Model file for the job. Use its own axes, mm. A direction names the side the tool comes from. Give positions to 0.01 mm unless a question says otherwise; leave off trailing zeros. Order: outer loops, then holes, each group sorted by start corner. A loop starts at its lowest first (then second) coordinate and runs counter-clockwise, first axis right, second up. Notation, with made-up numbers: (43, 52) -> (63, 52) arc R25 ccw to (63, 81) -> close; hole circle Ø9 at (18, -15.75). An arc over 180 degrees is marked (long way). Answer in a Markdown table with one row per item. Add a question column.
from build123d import *

# Parameters (mm, degrees)
SKETCH2_W           = 636
SKETCH2_H           = 753
BOSS_EXTRUDE1_DEPTH = 600
SKETCH3_W           = 600
SKETCH3_H           = 735
CUT_EXTRUDE1_DEPTH  = 600
BOSS_EXTRUDE2_START = -18
SKETCH4_W           = 600
SKETCH4_H           = 735
BOSS_EXTRUDE2_DEPTH = 9
BOSS_EXTRUDE3_START = -102
SKETCH5_W           = 636
SKETCH5_H           = 102
BOSS_EXTRUDE3_DEPTH = 18
SKETCH6_W           = 636
SKETCH6_H           = 102
BOSS_EXTRUDE4_DEPTH = 18
CUT_EXTRUDE2_REACH  = 1155.909
SKETCH7_W           = 600
SKETCH7_H           = 462


with BuildPart() as part:
    # Sketch2 → Boss-Extrude1 (new body)
    with BuildSketch(Plane.XY):
        with Locations((318, 376.5)):
            Rectangle(SKETCH2_W, SKETCH2_H)
    extrude(amount=BOSS_EXTRUDE1_DEPTH)

    # Sketch3 → Cut-Extrude1 (cut)
    with BuildSketch(Plane.XY.offset(600)):
        with Locations((318, 385.5)):
            Rectangle(SKETCH3_W, SKETCH3_H)
    extrude(amount=-CUT_EXTRUDE1_DEPTH, mode=Mode.SUBTRACT)

    # Sketch4 → Boss-Extrude2 (add)
    with BuildSketch(Plane(origin=(0, 0, 0), x_dir=(-1, 0, 0), z_dir=(0, 0, -1)).offset(BOSS_EXTRUDE2_START)):
        with Locations((-318, 385.5)):
            Rectangle(SKETCH4_W, SKETCH4_H)
    extrude(amount=BOSS_EXTRUDE2_DEPTH)

    # Sketch5 → Boss-Extrude3 (add)
    with BuildSketch(Plane.XY.offset(600).offset(BOSS_EXTRUDE3_START)):
        with Locations((318, -51)):
            Rectangle(SKETCH5_W, SKETCH5_H)
    extrude(amount=-BOSS_EXTRUDE3_DEPTH)

    # Sketch6 → Boss-Extrude4 (add)
    with BuildSketch(Plane(origin=(0, 0, 0), x_dir=(-1, 0, 0), z_dir=(0, 0, -1))):
        with Locations((-318, -51)):
            Rectangle(SKETCH6_W, SKETCH6_H)
    extrude(amount=-BOSS_EXTRUDE4_DEPTH)

    # Sketch7 → Cut-Extrude2 (cut, up to next)
    with BuildSketch(Plane.XZ, mode=Mode.PRIVATE) as cut_extrude2_sk1:
        with Locations((318, 249)):
            Rectangle(SKETCH7_W, SKETCH7_H)
    cut_extrude2_tool1 = extrude(cut_extrude2_sk1.sketch, amount=-CUT_EXTRUDE2_REACH, mode=Mode.PRIVATE) & part.part
    add(cut_extrude2_tool1.solids().sort_by_distance((318, 0, 249))[0], mode=Mode.SUBTRACT)


solid = part.part
Item 1: Which spindle directions (+Z, -Z, +X, -X, +Y, -Y) get a long thin tool onto all of the face, cutting with end or side? Do faces 4 (the flat face through (0, 320, 296)), 5 (the flat face through (314, 18, 541)), 6 (the flat face through (317, 16, 600)), 7 (the flat face through (314, -50, 498)), 8 (the flat face through (322, 391, 9)). Say none if no direction does.
Item 2: Saw through at D-D on y = 480.5. List the corners of the cut face in (x, z).
Item 3: Pin check, flat tips, straight feed: pin 1 Ø14.5 at (x, z) = (627, 300) entering from -Y; pin 2 Ø1 at (x, y) = (341.5, 269) entering from +Z; pin 3 Ø2 at (x, y) = (76, 134.5) entering from -Z. Stop position of each tip, or through.
Item 4: Saw through at C-C on x = 432. List the corners of the cut face in (y, z).
Item 5: Saw through at A-A on y = -20. List the corners of the cut face in (x, z), plus the area to 3 significant figures.
Item 6: Two-plate mould, pull along Z, no slides. Class faces 1 (the flat face through (296, 11, 0)), 2 (the flat face through (314, -41, 480)), 3 (the flat face through (636, 320, 296)): pulls with the +Z half, pulls with the -Z half, needs draft (parallel to the pull), parting line crosses it, or undercut.
Item 7: Wall check: line 1 (Z direction, x = 111, y = -40.5); line 2 (X direction, y = 302, z = 450); line 3 (Z direction, x = 60, y = 561.5). Give the ranges that are in metal, low to high.
Item 8: Saw through at B-B on z = 86.5. List the corners of the cut face in (x, y).
Evaluation:
| question | item | result |
|---|---|---|
| 1 | face 4 | +Z, -Z, -X, +Y, -Y |
| 1 | face 5 | +Z, +Y |
| 1 | face 6 | +Z, +X, -X, +Y, -Y |
| 1 | face 7 | +Z, +X, -X, -Y |
| 1 | face 8 | -Z, +Y |
| 2 | outline | (0, 0) -> (18, 0) -> (18, 9) -> (618, 9) -> (618, 0) -> (636, 0) -> (636, 600) -> (618, 600) -> (618, 18) -> (18, 18) -> (18, 600) -> (0, 600) -> close |
| 3 | pin 1 | stops at y = 0 |
| 3 | pin 2 | stops at z = 18 |
| 3 | pin 3 | stops at z = 9 |
| 4 | outline | (-102, 0) -> (18, 0) -> (18, 9) -> (753, 9) -> (753, 18) -> (-102, 18) -> close; (-102, 480) -> (18, 480) -> (18, 600) -> (0, 600) -> (0, 498) -> (-102, 498) -> close |
| 5 | outline | (0, 0) -> (636, 0) -> (636, 18) -> (0, 18) -> close; (0, 480) -> (636, 480) -> (636, 498) -> (0, 498) -> close |
| 5 | area | 22,900 mm2 |
| 6 | face 1 | pulls with the -Z half |
| 6 | face 2 | undercut |
| 6 | face 3 | needs draft |
| 7 | line 1 | z = 0 to 18, 480 to 498 |
| 7 | line 2 | x = 0 to 18, 618 to 636 |
| 7 | line 3 | z = 9 to 18 |
| 8 | outline | (0, 0) -> (18, 0) -> (18, 753) -> (0, 753) -> close; (618, 0) -> (636, 0) -> (636, 753) -> (618, 753) -> close |
